Source: CAD feature listing. Evaluate the final solid. Frame: model axes, mm. Round coordinates to 2 decimals unless told otherwise and drop trailing zeros. Answer in a Markdown table with one row per item.
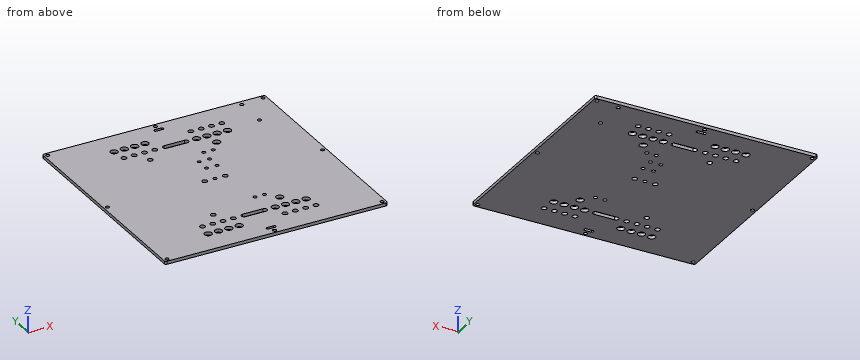
from build123d import *

# Parameters (mm, degrees)
SKETCH1_R           = 1.8
SKETCH1_R_2         = 3.57
SKETCH1_R_3         = 2.5
SKETCH1_R_4         = 1.75
BOSS_EXTRUDE1_DEPTH = 1.5


with BuildPart() as part:
    # Sketch1 → Boss-Extrude1 (new body, symmetric)
    with BuildSketch(Plane.XY):
        with BuildLine():
            Line((-106.25, -108), (106.25, -108))
            ThreePointArc((106.25, -108), (107.487436867, -107.487436867), (108, -106.25))
            Line((108, -106.25), (108, 106.25))
            ThreePointArc((108, 106.25), (107.487436867, 107.487436867), (106.25, 108))
            Line((106.25, 108), (-106.25, 108))
            ThreePointArc((-106.25, 108), (-107.487436867, 107.487436867), (-108, 106.25))
            Line((-108, 106.25), (-108, -106.25))
            ThreePointArc((-108, -106.25), (-107.487436867, -107.487436867), (-106.25, -108))
        make_face()
        with Locations((-104.5, 104.5)):
            Circle(SKETCH1_R, mode=Mode.SUBTRACT)
        with Locations((0, 104.5)):
            Circle(SKETCH1_R, mode=Mode.SUBTRACT)
        with Locations((104.5, 104.5)):
            Circle(SKETCH1_R, mode=Mode.SUBTRACT)
        with Locations((-104.5, 0)):
            Circle(SKETCH1_R, mode=Mode.SUBTRACT)
        Circle(SKETCH1_R, mode=Mode.SUBTRACT)
        with Locations((104.5, 0)):
            Circle(SKETCH1_R, mode=Mode.SUBTRACT)
        with Locations((-104.5, -104.5)):
            Circle(SKETCH1_R, mode=Mode.SUBTRACT)
        with Locations((0, -104.5)):
            Circle(SKETCH1_R, mode=Mode.SUBTRACT)
        with Locations((104.5, -104.5)):
            Circle(SKETCH1_R, mode=Mode.SUBTRACT)
        with Locations((-52.3, -82.65)):
            Circle(SKETCH1_R_2, mode=Mode.SUBTRACT)
        with Locations((-42.3, -82.65)):
            Circle(SKETCH1_R_2, mode=Mode.SUBTRACT)
        with Locations((-32.3, -82.65)):
            Circle(SKETCH1_R_2, mode=Mode.SUBTRACT)
        with Locations((-22.3, -82.65)):
            Circle(SKETCH1_R_2, mode=Mode.SUBTRACT)
        with Locations((-50.32, -69)):
            Circle(SKETCH1_R_3, mode=Mode.SUBTRACT)
        with Locations((-40.32, -69)):
            Circle(SKETCH1_R_3, mode=Mode.SUBTRACT)
        with Locations((-30.32, -69)):
            Circle(SKETCH1_R_3, mode=Mode.SUBTRACT)
        with Locations((-20.32, -69)):
            Circle(SKETCH1_R_3, mode=Mode.SUBTRACT)
        with Locations((42.3, -82.65)):
            Circle(SKETCH1_R_3, mode=Mode.SUBTRACT)
        with Locations((32.3, -82.65)):
            Circle(SKETCH1_R_3, mode=Mode.SUBTRACT)
        with Locations((22.3, -82.65)):
            Circle(SKETCH1_R_3, mode=Mode.SUBTRACT)
        with Locations((52.3, -82.65)):
            Circle(SKETCH1_R_3, mode=Mode.SUBTRACT)
        with Locations((50.32, -69)):
            Circle(SKETCH1_R_2, mode=Mode.SUBTRACT)
        with Locations((40.32, -69)):
            Circle(SKETCH1_R_2, mode=Mode.SUBTRACT)
        with Locations((30.32, -69)):
            Circle(SKETCH1_R_2, mode=Mode.SUBTRACT)
        with Locations((20.32, -69)):
            Circle(SKETCH1_R_2, mode=Mode.SUBTRACT)
        with Locations((-32.3, -55.35)):
            Circle(SKETCH1_R_3, mode=Mode.SUBTRACT)
        with Locations((32.3, -55.35)):
            Circle(SKETCH1_R_2, mode=Mode.SUBTRACT)
        with Locations((14, -45)):
            Circle(SKETCH1_R, mode=Mode.SUBTRACT)
        with Locations((23.12, -45)):
            Circle(SKETCH1_R, mode=Mode.SUBTRACT)
        with Locations((-10, 0)):
            Circle(SKETCH1_R_3, mode=Mode.SUBTRACT)
        with Locations((10, 0)):
            Circle(SKETCH1_R_3, mode=Mode.SUBTRACT)
        with Locations((2.5, 32.3)):
            Circle(SKETCH1_R_4, mode=Mode.SUBTRACT)
        with Locations((12.64, 32.3)):
            Circle(SKETCH1_R_4, mode=Mode.SUBTRACT)
        with Locations((2.5, 19.47)):
            Circle(SKETCH1_R_4, mode=Mode.SUBTRACT)
        with Locations((12.64, 19.47)):
            Circle(SKETCH1_R_4, mode=Mode.SUBTRACT)
        with Locations((23.12, 45)):
            Circle(SKETCH1_R, mode=Mode.SUBTRACT)
        with Locations((14, 45)):
            Circle(SKETCH1_R, mode=Mode.SUBTRACT)
        with Locations((32.3, 55.35)):
            Circle(SKETCH1_R_2, mode=Mode.SUBTRACT)
        with Locations((-32.3, 55.35)):
            Circle(SKETCH1_R_3, mode=Mode.SUBTRACT)
        with Locations((20.32, 69)):
            Circle(SKETCH1_R_2, mode=Mode.SUBTRACT)
        with Locations((30.32, 69)):
            Circle(SKETCH1_R_2, mode=Mode.SUBTRACT)
        with Locations((40.32, 69)):
            Circle(SKETCH1_R_2, mode=Mode.SUBTRACT)
        with Locations((50.32, 69)):
            Circle(SKETCH1_R_2, mode=Mode.SUBTRACT)
        with Locations((52.3, 82.65)):
            Circle(SKETCH1_R_3, mode=Mode.SUBTRACT)
        with Locations((22.3, 82.65)):
            Circle(SKETCH1_R_3, mode=Mode.SUBTRACT)
        with Locations((32.3, 82.65)):
            Circle(SKETCH1_R_3, mode=Mode.SUBTRACT)
        with Locations((42.3, 82.65)):
            Circle(SKETCH1_R_3, mode=Mode.SUBTRACT)
        with Locations((-20.32, 69)):
            Circle(SKETCH1_R_3, mode=Mode.SUBTRACT)
        with Locations((-30.32, 69)):
            Circle(SKETCH1_R_3, mode=Mode.SUBTRACT)
        with Locations((-40.32, 69)):
            Circle(SKETCH1_R_3, mode=Mode.SUBTRACT)
        with Locations((-50.32, 69)):
            Circle(SKETCH1_R_3, mode=Mode.SUBTRACT)
        with Locations((-22.3, 82.65)):
            Circle(SKETCH1_R_2, mode=Mode.SUBTRACT)
        with Locations((-32.3, 82.65)):
            Circle(SKETCH1_R_2, mode=Mode.SUBTRACT)
        with Locations((-42.3, 82.65)):
            Circle(SKETCH1_R_2, mode=Mode.SUBTRACT)
        with Locations((-52.3, 82.65)):
            Circle(SKETCH1_R_2, mode=Mode.SUBTRACT)
        with Locations((83, 103)):
            Circle(SKETCH1_R, mode=Mode.SUBTRACT)
        with Locations((83, 72)):
            Circle(SKETCH1_R, mode=Mode.SUBTRACT)
        with BuildLine():
            Line((-3.25, -97.12), (3.25, -97.12))
            ThreePointArc((3.25, -97.12), (4.75, -98.62), (3.25, -100.12))
            Line((3.25, -100.12), (-3.25, -100.12))
            ThreePointArc((-3.25, -100.12), (-4.75, -98.62), (-3.25, -97.12))
        make_face(mode=Mode.SUBTRACT)
        with BuildLine():
            Line((-10, -66.5), (10, -66.5))
            ThreePointArc((10, -66.5), (12.5, -69), (10, -71.5))
            Line((10, -71.5), (-10, -71.5))
            ThreePointArc((-10, -71.5), (-12.5, -69), (-10, -66.5))
        make_face(mode=Mode.SUBTRACT)
        with BuildLine():
            Line((-3.25, 97.12), (3.25, 97.12))
            ThreePointArc((3.25, 97.12), (4.75, 98.62), (3.25, 100.12))
            Line((3.25, 100.12), (-3.25, 100.12))
            ThreePointArc((-3.25, 100.12), (-4.75, 98.62), (-3.25, 97.12))
        make_face(mode=Mode.SUBTRACT)
        with BuildLine():
            Line((-10, 66.5), (10, 66.5))
            ThreePointArc((10, 66.5), (12.5, 69), (10, 71.5))
            Line((10, 71.5), (-10, 71.5))
            ThreePointArc((-10, 71.5), (-12.5, 69), (-10, 66.5))
        make_face(mode=Mode.SUBTRACT)
    extrude(amount=BOSS_EXTRUDE1_DEPTH, both=True)


solid = part.part
Q1. Section A-A (z = 0.6). State how many separate pieces and enclosed holes the cut face has, and give its area (3 significant figures).
Solutions:
| item | result |
|---|---|
| separate pieces | 1 |
| enclosed holes | 61 |
| area | 45,100 mm2 |
Q2. Contact query for flat-ended pins moving along their axis: pin 1 Ø6 at (x, y) = (22.3, -82.65) entering from +Z; pin 2 Ø6.5 at (x, y) = (30.32, 69) entering from +Z. Output: stop coordinate, or through.
Solutions:
| item | result |
|---|---|
| pin 1 | stops at z = 1.5 |
| pin 2 | passes through |
Q3. Material intervals for probe 1 along Y at (x, z) = (104.5, -0.3); probe 2 along X at (y, z) = (32, -1.25); probe 3 along Y at (x, z) = (-43, -0.4), sorted ascending.
Solutions:
| item | result |
|---|---|
| probe 1 | y = -108 to -106.3, -102.7 to -1.8, 1.8 to 102.7, 106.3 to 108 |
| probe 2 | x = -108 to 0.78, 4.22 to 10.92, 14.36 to 108 |
| probe 3 | y = -108 to -86.15, -79.15 to 79.15, 86.15 to 108 |
